Part model, mm, in its own coordinate system. A direction names the side the tool comes from. Round coordinates to 2 decimals unless told otherwise and drop trailing zeros. Loops run counter-clockwise (first coordinate to the right, second up) from the corner with the lowest first, then second, coordinate; pieces in that order, holes last. Notation, with made-up numbers: (57.25, 14) -> (79.25, 14) arc R19 cw to (79.25, 23) -> close; hole circle Ø8 at (76, 71). An arc over 180 degrees is marked (long way). Answer as CSV lines item,"result".
from build123d import *

# Parameters (mm, degrees)
F1_DEPTH      = 38
F1_DEPTH_BACK = 38
F3_DEPTH      = 1555.001
F4_R          = 2


with BuildPart() as f1:
    # F0 (on Right) → F1 (new body, two sides)
    with BuildSketch(Plane.YZ) as f1_sk:
        Polygon((-777.5, -11), (777.5, -11), (777.5, -8), (727.5, -8), (727.5, 11), (-727.5, 11), (-727.5, -8), (-777.5, -8), align=None)
    extrude(amount=F1_DEPTH)
    extrude(f1_sk.sketch, amount=-F1_DEPTH_BACK)

    # F2 (on face) → F3 (cut, through all)
    with BuildSketch(Plane.XZ.offset(777.5)):
        with BuildLine():
            Line((-36.4364916731, -8), (36.4364916731, -8))
            ThreePointArc((36.4364916731, -8), (36.4840593925, -7.752008585), (36.5, -7.5))
            Line((36.5, -7.5), (36.5, 7.5))
            ThreePointArc((36.5, 7.5), (35.9142135624, 8.9142135624), (34.5, 9.5))
            Line((34.5, 9.5), (-34.5, 9.5))
            ThreePointArc((-34.5, 9.5), (-35.9142135624, 8.9142135624), (-36.5, 7.5))
            Line((-36.5, 7.5), (-36.5, -7.5))
            ThreePointArc((-36.5, -7.5), (-36.4840593925, -7.752008585), (-36.4364916731, -8))
        make_face()
        with BuildLine():
            Line((-34.5, -9.5), (34.5, -9.5))
            ThreePointArc((34.5, -9.5), (35.7247448714, -9.0811388301), (36.4364916731, -8))
            Line((36.4364916731, -8), (-36.4364916731, -8))
            ThreePointArc((-36.4364916731, -8), (-35.7247448714, -9.0811388301), (-34.5, -9.5))
        make_face()
    extrude(amount=-F3_DEPTH, mode=Mode.SUBTRACT)

    # F4
    f4_edges = [f1.edges().sort_by_distance(p)[0] for p in [
        (-38, 0, 11),
        (-38, 0, -11),
        (38, 0, -11),
        (38, 0, 11),
    ]]
    fillet(f4_edges, radius=F4_R)


solid = f1.part
Q1. Saw through at A-A, the plane z = -2.5. Write the cut outline in (x, y).
Geometry results:
outline,"(-38, -727.5) -> (-36.5, -727.5) -> (-36.5, 727.5) -> (-38, 727.5) -> close; (36.5, -727.5) -> (38, -727.5) -> (38, 727.5) -> (36.5, 727.5) -> close"
Q2. Saw through at C-C, the plane y = -648. Write the cut outline in (x, z).
Geometry results:
outline,"(-38, -9) arc R2 ccw to (-36, -11) -> (36, -11) arc R2 ccw to (38, -9) -> (38, 9) arc R2 ccw to (36, 11) -> (-36, 11) arc R2 ccw to (-38, 9) -> close; hole (-36.5, -7.5) arc R2 ccw to (-34.5, -9.5) -> (34.5, -9.5) arc R2 ccw to (36.5, -7.5) -> (36.5, 7.5) arc R2 ccw to (34.5, 9.5) -> (-34.5, 9.5) arc R2 ccw to (-36.5, 7.5) -> close"
Q3. Saw through at B-B, the plane x = -17. Write the cut outline in (y, z), then the cut area to 4 significant figures.
Geometry results:
outline,"(-777.5, -11) -> (777.5, -11) -> (777.5, -9.5) -> (-777.5, -9.5) -> close; (-727.5, 9.5) -> (727.5, 9.5) -> (727.5, 11) -> (-727.5, 11) -> close"
area,"4,515 mm2"
Q4. Drop flat-ended pins along their axis: P1, Ø0.5, axis at x = 37, y = 746.5, coming from the +Z side; P2, Ø9.5, axis at x = 1, z = 5.5, coming from the -Y side. Give the stop position or say it passes through.
Geometry results:
P1,"z = -8"
P2,"y = -727.5"
Q5. Drill centre lines: line 1 along Z through (x, y) = (-15, 455); line 2 along X through (y, z) = (550, -6); line 3 along X through (y, z) = (474, 8.25). Where is each one in solid material? Low to high.
Geometry results:
line 1,"-11 to -9.5, 9.5 to 11"
line 2,"-38 to -36.5, 36.5 to 38"
line 3,"-38 to -36.35, 36.35 to 38"
Q6. Which spindle directions (+Z, -Z, +X, -X, +Y, -Y) get a long thin tool onto all of the face, cutting with end or side? Do faces 1 (the face through (1, 10, 11)), 2 (the face through (0, -11, -9.5)). Say none if no direction does.
Geometry results:
face 1,"+Z, +X, -X, +Y, -Y"
face 2,"+Y, -Y"
